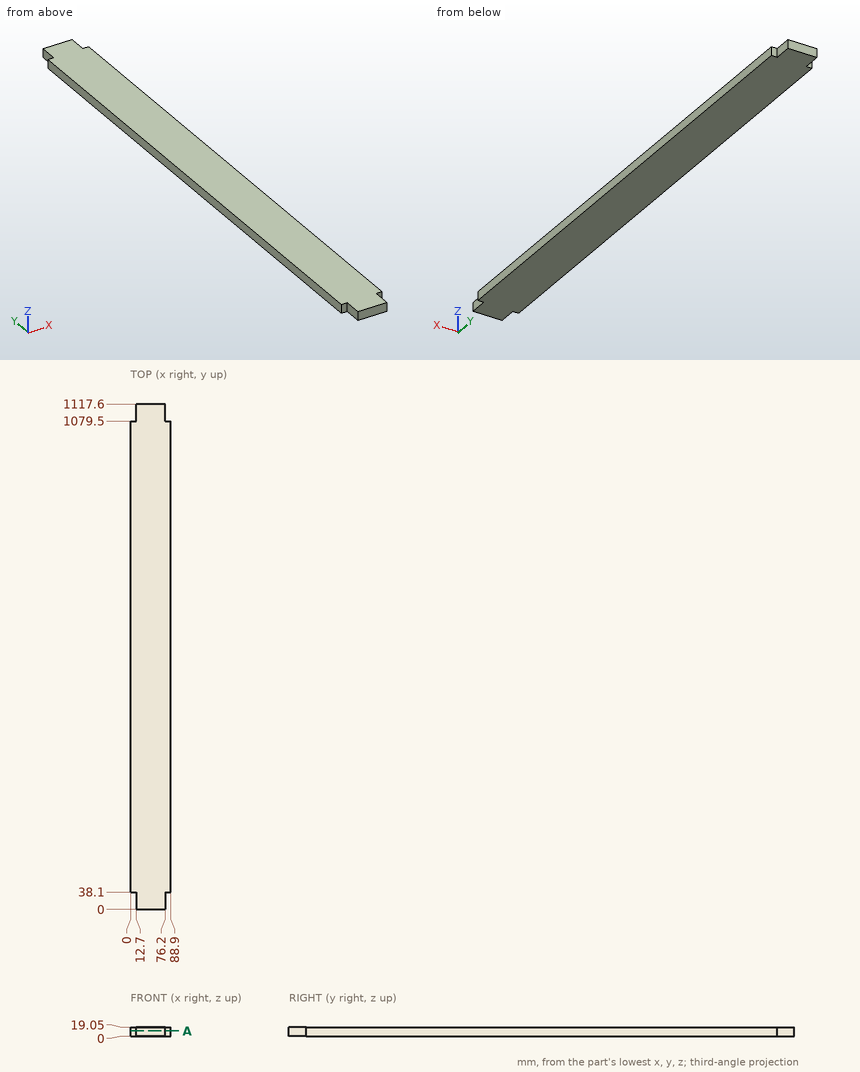
Can you work these out from the drawing? Everything is in mm from the part's minimum corner. Give positions to 0.01 mm unless a question says otherwise; leave off trailing zeros. Loops run counter-clockwise (first coordinate to the right, second up) from the corner with the lowest first, then second, coordinate; pieces in that order, holes last. Notation, with made-up numbers: (73, 33) -> (119, 33) arc R21 cw to (119, 42) -> close; hole circle Ø9 at (5.25, -30). An arc over 180 degrees is marked (long way). Write item = value, one per line.
1) Suppose I cut it at A-A on z = 11.5. Write out the boundary of the cut face in (x, y).
Check result:
outline = (0, 38.1) -> (12.7, 38.1) -> (12.7, 0) -> (76.2, 0) -> (76.2, 38.1) -> (88.9, 38.1) -> (88.9, 1079.5) -> (76.2, 1079.5) -> (76.2, 1117.6) -> (12.7, 1117.6) -> (12.7, 1079.5) -> (0, 1079.5) -> close
2) I need wall thicknesses on L1, parallel to Y at x = 82.5, z = 13.5. Which ranges of the line are inside material? Lowest first, please. Write a range as from..to.
Check result:
L1 = 38.1..1079.5
3) Will these pins go through, and if not, where does the flat tip stop? pin 1 (5 mm diameter, centred on x = 69.5, y = 176, fed in from -Z); pin 2 (10 mm diameter, centred on x = 5.5, z = 7, fed in from +Y); pin 3 (5.5 mm diameter, centred on y = 1103.5, z = 13.5, fed in from -X); pin 4 (10 mm diameter, centred on x = 83, z = 11.5, fed in from -Y).
Check result:
pin_1 = 0
pin_2 = 1079.5
pin_3 = 12.7
pin_4 = 38.1
